```python
from build123d import *

# Parameters (mm, degrees)
BOSS_EXTRUDE1_DEPTH      = 25
BOSS_EXTRUDE1_DEPTH_BACK = 25
SKETCH3_R                = 11.05
SKETCH3_R_2              = 1.75
CUT_EXTRUDE1_DEPTH       = 78.723870207
CUT_EXTRUDE2_DEPTH       = 78.723870207
CHAMFER1_SIZE            = 5
FILLET1_R                = 2
FILLET2_R                = 3.5
BOSS_EXTRUDE2_DEPTH      = 2.5


with BuildPart() as part:
    # Sketch1 → Boss-Extrude1 (new, two sides: drawn at the far end of the back side and taken through both)
    with BuildSketch(Plane(origin=(0, 0, 0), x_dir=(0, 0, -1), z_dir=(1, 0, 0)).offset(-BOSS_EXTRUDE1_DEPTH_BACK)):
        Polygon((-50, 0), (-50, -2.8), (-2.8, -2.8), (-2.8, -54), (0, -54), (0, 0), align=None)
    extrude(amount=BOSS_EXTRUDE1_DEPTH + BOSS_EXTRUDE1_DEPTH_BACK)

    # Sketch3 → Cut-Extrude1 (cut, through all)
    with BuildSketch(Plane(origin=(0, 0, 0), x_dir=(1, 0, 0), z_dir=(0, 1, 0))):
        with Locations(Location((0, -29, 0), (0, 0, 270))):
            Circle(SKETCH3_R)
        with Locations(Location((-15.5, -13.5, 0), (0, 0, 270))):
            Circle(SKETCH3_R_2)
        with Locations(Location((15.5, -13.5, 0), (0, 0, 270))):
            Circle(SKETCH3_R_2)
        with Locations(Location((15.5, -44.5, 0), (0, 0, 270))):
            Circle(SKETCH3_R_2)
        with Locations(Location((-15.5, -44.5, 0), (0, 0, 270))):
            Circle(SKETCH3_R_2)
    extrude(amount=-CUT_EXTRUDE1_DEPTH, mode=Mode.SUBTRACT)

    # Sketch4 → Cut-Extrude2 (cut, through all)
    with BuildSketch(Plane(origin=(0, 0, 0), x_dir=(-1, 0, 0), z_dir=(0, 0, -1))):
        with BuildLine():
            Line((-17.1, -43), (-17.1, -13))
            ThreePointArc((-17.1, -13), (-15, -10.9), (-12.9, -13))
            Line((-12.9, -13), (-12.9, -43))
            ThreePointArc((-12.9, -43), (-15, -45.1), (-17.1, -43))
        make_face()
        with BuildLine():
            Line((12.9, -43), (12.9, -13))
            ThreePointArc((12.9, -13), (15, -10.9), (17.1, -13))
            Line((17.1, -13), (17.1, -43))
            ThreePointArc((17.1, -43), (15, -45.1), (12.9, -43))
        make_face()
    extrude(amount=-CUT_EXTRUDE2_DEPTH, mode=Mode.SUBTRACT)

    # Chamfer1
    chamfer1_edges = [part.edges().sort_by_distance(p)[0] for p in [
        (25, -1.4, 50),
        (25, -54, 1.4),
        (-25, -54, 1.4),
        (-25, -1.4, 50),
    ]]
    chamfer(chamfer1_edges, length=CHAMFER1_SIZE)

    # Fillet1
    fillet1_edges = [part.edges().sort_by_distance(p)[0] for p in [
        (0, -2.8, 2.8),
    ]]
    fillet(fillet1_edges, radius=FILLET1_R)

    # Fillet2
    fillet2_edges = [part.edges().sort_by_distance(p)[0] for p in [
        (0, 0, 0),
    ]]
    fillet(fillet2_edges, radius=FILLET2_R)

    # Sketch5 → Boss-Extrude2 (add)
    with BuildSketch(Plane.ZY.offset(25)):
        Polygon((2.8, -5.3), (5.3, -2.8), (22, -2.8), (2.8, -16), align=None)
    boss_extrude2 = extrude(amount=-BOSS_EXTRUDE2_DEPTH)

    # Mirror1: Boss-Extrude2 across plane
    add(boss_extrude2.mirror(Plane(origin=(0, 0, 0), x_dir=(0, 0, 1), z_dir=(1, 0, 0))))


solid = part.part
```
Check sheet for the modelled part. Datum: model origin and axes. Units: mm. A direction names the side the tool comes from. Coordinates: 2 decimals unless noted, no trailing zeros. Write each loop counter-clockwise with the first axis right and the second up, starting at its lowest first coordinate (ties: lowest second). Pieces come first, ordered by that corner, then holes. Notation, with made-up numbers: (71.5, 72.5) -> (90.5, 72.5) arc R13 cw to (90.5, 97.5) -> close; hole circle Ø6 at (11, 18.5). An arc over 180 degrees is marked (long way). Use a Markdown table: item, result.
1. Sectioned sample at A-A (z = 29). Enter the section's corners in (x, y).
Reported:
| item | result |
|---|---|
| outline | (-25, -2.8) -> (-11.05, -2.8) -> (-11.05, 0) -> (-25, 0) -> close; (11.05, -2.8) -> (25, -2.8) -> (25, 0) -> (11.05, 0) -> close |
2. Tool access check on faces 5 (the flat face through (22, -52, 1)), 6 (the cylindrical face through (15, -10.9, 1.4)), 7 (the flat face through (22.5, -6, 8)). Record the directions out of +Z, -Z, +X, -X, +Y, -Y that give a thin tool (end or side, any length) a straight path to the whole face; none if there is none.
Reported:
| item | result |
|---|---|
| face 5 | +Z, -Z, +X, -Y |
| face 6 | +Z, -Z |
| face 7 | +Z, -Y |
3. Sectioned sample at D-D (z = 14). Enter the section's corners in (x, y).
Reported:
| item | result |
|---|---|
| outline | (-25, -8.3) -> (-22.5, -8.3) -> (-22.5, -2.8) -> (-17.18, -2.8) -> (-17.18, 0) -> (-25, 0) -> close; (-13.82, -2.8) -> (13.82, -2.8) -> (13.82, 0) -> (-13.82, 0) -> close; (17.18, -2.8) -> (22.5, -2.8) -> (22.5, -8.3) -> (25, -8.3) -> (25, 0) -> (17.18, 0) -> close |
4. Go/stop test with flat-tipped pins: pin 1 Ø4.5 at (x, z) = (-15.5, 13.5) entering from +Y; pin 2 Ø6 at (x, y) = (11.5, -24) entering from +Z; pin 3 Ø5.5 at (x, z) = (15.5, 44.5) entering from -Y. Record where each tip stops, or that it passes through.
Reported:
| item | result |
|---|---|
| pin 1 | stops at y = 0 |
| pin 2 | stops at z = 2.8 |
| pin 3 | stops at y = -2.8 |
5. Sectioned sample at C-C (y = -34.5). Enter the section's corners in (x, z), plus the area to 3 significant figures.
Reported:
| item | result |
|---|---|
| outline | (-25, 0) -> (-17.1, 0) -> (-17.1, 2.8) -> (-25, 2.8) -> close; (-12.9, 0) -> (12.9, 0) -> (12.9, 2.8) -> (-12.9, 2.8) -> close; (17.1, 0) -> (25, 0) -> (25, 2.8) -> (17.1, 2.8) -> close |
| area | 116 mm2 |
6. Sectioned sample at B-B (x = 0). Enter the section's corners in (y, z), plus the area to 3 significant figures.
Reported:
| item | result |
|---|---|
| outline | (-54, 0) -> (-3.5, 0) arc R3.5 ccw to (0, 3.5) -> (0, 17.95) -> (-2.8, 17.95) -> (-2.8, 4.8) arc R2 cw to (-4.8, 2.8) -> (-54, 2.8) -> close; (-2.8, 40.05) -> (0, 40.05) -> (0, 50) -> (-2.8, 50) -> close |
| area | 220 mm2 |
7. Scan lines: line 1 along X through (y, z) = (-1, 44.5); line 2 along Z through (x, y) = (-15, -1); line 3 along X through (y, z) = (-0.9, 29). Record each from-to range of solid material in increasing order.
Reported:
| item | result |
|---|---|
| line 1 | x = -25 to -17.25, -13.75 to 13.75, 17.25 to 25 |
| line 2 | z = 1.05 to 11.82, 15.18 to 42.82, 46.18 to 50 |
| line 3 | x = -25 to -11.05, 11.05 to 25 |
8. Release check for a two-part mould opening along Z. For faces 1 (the cylindrical face through (17.235, -1.38, 13.272)), 2 (the flat face through (-22.5, -6, 8)), 3 (the cylindrical face through (-14, -1.4, 14.4)), 4 (the flat face through (0, -29, 0)) record: pulls with the +Z half, pulls with the -Z half, needs draft (parallel to the pull), parting line crosses it, or undercut.
Reported:
| item | result |
|---|---|
| face 1 | undercut |
| face 2 | needs draft |
| face 3 | undercut |
| face 4 | pulls with the -Z half |
